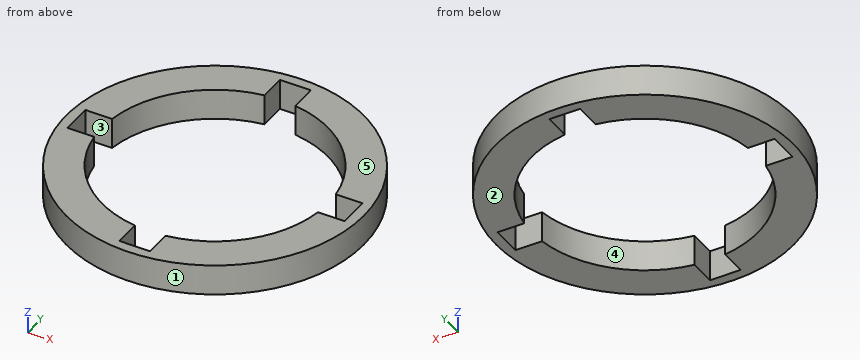
Autodesk Inventor part; units mm, degrees
ref_plane "YZ Plane" through (0, 0, 0) normal (1, 0, 0) x (0, 1, 0)
ref_plane "XZ Plane" through (0, 0, 0) normal (0, 1, 0) x (-1, 0, 0)
ref_plane "XY Plane" through (0, 0, 0) normal (0, 0, 1) x (1, 0, 0)
sketch "Sketch1" plane through (0, 0, 0) normal (0, 0, 1) x (1, 0, 0)
  line L0 (-25, -3) -> (-25, 3)
  line L1 (17, -3) -> (17, 3)
  line L2 (-25, -3) -> (-31, -3)
  line L3 (-31, -3) -> (-31, 3)
  line L4 (-31, 3) -> (-25, 3)
  line L5 (-25, 3) -> (-25, -3)
  line L6 (17, -3) -> (23, -3)
  line L7 (23, -3) -> (23, 3)
  line L8 (23, 3) -> (17, 3)
  line L9 (17, 3) -> (17, -3)
  circle A0 centre (-4, 0) radius 29
  line L10 (-1, -21) -> (-1, -27)
  line L11 (-1, -27) -> (-7, -27)
  line L12 (-7, -27) -> (-7, -21)
  line L13 (-7, -21) -> (-1, -21)
  line L14 (17, 3) -> (23, 3)
  line L15 (23, 3) -> (23, -3)
  line L16 (23, -3) -> (17, -3)
  line L17 (17, -3) -> (17, 3)
  line L18 (-7, 21) -> (-7, 27)
  line L19 (-7, 27) -> (-1, 27)
  line L20 (-1, 27) -> (-1, 21)
  line L21 (-1, 21) -> (-7, 21)
  circle A1 centre (-4, 0) radius 22
  line L22 (-4, 0) -> (17, 0)
  point P0 (-7, -21)
  point P1 (-1, 21)
  dimension "d10" = 6
  dimension "d12" = 6
  dimension "d21" = 360
  dimension "d25" = 44
  dimension "d29" = 21
  dimension "d30" = 21
extrude "Extrusion1" add sketch "Sketch1" along normal blind 6
Model file for the job. Use its own axes, mm. Face numbers are marked on the shaded views. A direction names the side the tool comes from. Give positions to 0.01 mm unless a question says otherwise; leave off trailing zeros. Loops run counter-clockwise (first coordinate to the right, second up) from the corner with the lowest first, then second, coordinate; pieces in that order, holes last. Notation, with made-up numbers: (33, -11.75) -> (81, -11.75) arc R13 ccw to (81, 8.25) -> close; hole circle Ø11 at (-14, -10.5). An arc over 180 degrees is marked (long way). Use a Markdown table: item, result. Add a question column.
(1) Slice it at B-B on z = 1.2. List the corners of the cut face in (x, y), and give its area (4 significant figures).
(2) Slice it at A-A on x = -4. List the corners of the cut face in (y, z).
(3) Slice it at C-C on y = 0. List the corners of the cut face in (x, z).
(4) Wall check: line 1 along X through (y, z) = (0.5, 3.5); line 2 along Y through (x, z) = (-4.5, 1.2); line 3 along X through (y, z) = (10.5, 1.6). Give the ranges that are in metal, low to high.
(5) Drop flat-ended pins along their axis: pin 1 Ø1.6 at (y, z) = (-25.5, 3) entering from -X; pin 2 Ø3 at (x, z) = (-3.5, 1.5) entering from -Y; pin 3 Ø2.5 at (x, z) = (19.5, 1.5) entering from +Y. Give the stop position or say it passes through.
(6) Tool access for the marked faces 4 and 5: list every direction of +Z, -Z, +X, -X, +Y, -Y with a clear straight run to the whole face (end or side of a thin tool).
(7) Mould opens along X. For the marked faces 1, 2 and 3 say: +X half, -X half, draft (parallel to the pull), parting line (faces both ways), or undercut.
Filled sheet:
| question | item | result |
|---|---|---|
| 1 | outline | circle Ø58 at (-4, 0); hole (-31, -3) -> (-25.79, -3) arc R22 ccw to (-7, -21.79) -> (-7, -27) -> (-1, -27) -> (-1, -21.79) arc R22 ccw to (17.79, -3) -> (23, -3) -> (23, 3) -> (17.79, 3) arc R22 ccw to (-1, 21.79) -> (-1, 27) -> (-7, 27) -> (-7, 21.79) arc R22 ccw to (-25.79, 3) -> (-31, 3) -> close |
| 1 | area | 1,000 mm2 |
| 2 | outline | (-29, 0) -> (-27, 0) -> (-27, 6) -> (-29, 6) -> close; (27, 0) -> (29, 0) -> (29, 6) -> (27, 6) -> close |
| 3 | outline | (-33, 0) -> (-31, 0) -> (-31, 6) -> (-33, 6) -> close; (23, 0) -> (25, 0) -> (25, 6) -> (23, 6) -> close |
| 4 | line 1 | -33 to -31, 23 to 25 |
| 4 | line 2 | -29 to -27, 27 to 29 |
| 4 | line 3 | -31.03 to -23.33, 15.33 to 23.03 |
| 5 | pin 1 | x = -19.2 |
| 5 | pin 2 | y = -29 |
| 5 | pin 3 | y = 18.6 |
| 6 | face 4 | +Z, -Z |
| 6 | face 5 | +Z, +X, -X, +Y, -Y |
| 7 | face 1 | parting line |
| 7 | face 2 | draft |
| 7 | face 3 | undercut |
